from build123d import *

# Parameters (mm, degrees)
SKIZZE1_W                        = 17
SKIZZE1_H                        = 17
SKIZZE1_W_2                      = 16
SKIZZE1_H_2                      = 16
AUFSATZ_LINEAR_AUSTRAGEN1_DEPTH  = 19.7
SKIZZE10_W                       = 13.3
SKIZZE10_H                       = 20
AUFSATZ_LINEAR_AUSTRAGEN5_DEPTH  = 0.5
SKIZZE11_W                       = 5.3
SKIZZE11_H                       = 13.320508076
SCHNITT_LINEAR_AUSTRAGEN14_DEPTH = 11.433012702
AUFSATZ_LINEAR_AUSTRAGEN6_DEPTH  = 4
AUFSATZ_LINEAR_AUSTRAGEN7_DEPTH  = 4


with BuildPart() as part:
    # Skizze1 → Aufsatz-Linear austragen1 (new body)
    with BuildSketch(Plane(origin=(0, 0, 0), x_dir=(1, 0, 0), z_dir=(0, 1, 0))):
        Rectangle(SKIZZE1_W, SKIZZE1_H)
        Rectangle(SKIZZE1_W_2, SKIZZE1_H_2, mode=Mode.SUBTRACT)
    extrude(amount=AUFSATZ_LINEAR_AUSTRAGEN1_DEPTH)

    # Skizze10 → Aufsatz-Linear austragen5 (add)
    with BuildSketch(Plane(origin=(-2.530350227, 1.460898385, 0), x_dir=(0, 0, -1), z_dir=(0.866025404, -0.5, 0))):
        with Locations((-0.00194728, 31.060700455)):
            Rectangle(SKIZZE10_W, SKIZZE10_H)
    aufsatz_linear_austragen5 = extrude(amount=AUFSATZ_LINEAR_AUSTRAGEN5_DEPTH)

    # Skizze11 → Schnitt-Linear austragen14 (cut, through all)
    with BuildSketch(Plane.ZY.offset(-8)):
        with Locations((0.00194728, 26.360254038)):
            Rectangle(SKIZZE11_W, SKIZZE11_H)
    schnitt_linear_austragen14 = extrude(amount=-SCHNITT_LINEAR_AUSTRAGEN14_DEPTH, mode=Mode.SUBTRACT)

    # Skizze12 → Aufsatz-Linear austragen6 (add)
    with BuildSketch(Plane.XY.offset(6.65194728)):
        Polygon((18.433012702, 36.770508076), (8.5, 0), (8.5, 19.7), align=None)
    aufsatz_linear_austragen6 = extrude(amount=-AUFSATZ_LINEAR_AUSTRAGEN6_DEPTH)

    # Skizze13 → Aufsatz-Linear austragen7 (add)
    with BuildSketch(Plane(origin=(0, 0, -6.64805272), x_dir=(-1, 0, 0), z_dir=(0, 0, -1))):
        Polygon((-18.433012702, 36.770508076), (-8.5, 19.7), (-8.5, 0), align=None)
    aufsatz_linear_austragen7 = extrude(amount=-AUFSATZ_LINEAR_AUSTRAGEN7_DEPTH)

    # Spiegeln6: Aufsatz-Linear austragen5, Schnitt-Linear austragen14, Aufsatz-Linear austragen6, Aufsatz-Linear austragen7 across plane
    add(aufsatz_linear_austragen5.mirror(Plane(origin=(0, 0, 0), x_dir=(0, 0, 1), z_dir=(1, 0, 0))))
    add(schnitt_linear_austragen14.mirror(Plane(origin=(0, 0, 0), x_dir=(0, 0, 1), z_dir=(1, 0, 0))), mode=Mode.SUBTRACT)
    add(aufsatz_linear_austragen6.mirror(Plane(origin=(0, 0, 0), x_dir=(0, 0, 1), z_dir=(1, 0, 0))))
    add(aufsatz_linear_austragen7.mirror(Plane(origin=(0, 0, 0), x_dir=(0, 0, 1), z_dir=(1, 0, 0))))


solid = part.part
For this review, take the finished solid that the model builds, in its own axes (mm). A direction names the side the tool comes from. Give positions to 0.01 mm unless a question says otherwise; leave off trailing zeros. Order: outer loops, then holes, each group sorted by start corner. A loop starts at its lowest first (then second) coordinate and runs counter-clockwise, first axis right, second up. Notation, with made-up numbers: (54, -25.5) -> (102, -25.5) arc R19 cw to (102, -12.5) -> close; hole circle Ø1 at (-32.5, -18.5). An arc over 180 degrees is marked (long way). Write item = value, one per line.
1) We need section B-B, the plane z = -5. Give the boundary of the cut face in (x, y).
Findings:
outline = (-18.43, 36.77) -> (-8.5, 0) -> (-8, 0) -> (-8, 19.7) -> (-18, 37.02) -> close; (8, 0) -> (8.5, 0) -> (18.43, 36.77) -> (18, 37.02) -> (8, 19.7) -> close
2) Insertion check: pin 1 (6 mm diameter, centred on x = -8.5, y = 23, fed in from -Z); pin 2 (10 mm diameter, centred on y = 7, z = 5, fed in from -X); pin 3 (0.6 mm diameter, centred on x = 8.5, z = 0, fed in from +Y). Each pin has a flat end and moves straight along its axis. Give the tip position at first contact, or say it passes through.
Findings:
pin_1 = -6.65
pin_2 = -11.74
pin_3 = 19.7
3) We need section A-A, the plane z = -2. Give the boundary of the cut face in (x, y), and give its area (3 significant figures).
Findings:
outline = (-18.43, 36.77) -> (-16.27, 33.02) -> (-15.69, 33.02) -> (-18, 37.02) -> close; (-8.58, 19.7) -> (-8.5, 19.57) -> (-8.5, 0) -> (-8, 0) -> (-8, 19.7) -> close; (8, 0) -> (8.5, 0) -> (8.5, 19.57) -> (8.58, 19.7) -> (8, 19.7) -> close; (15.69, 33.02) -> (16.27, 33.02) -> (18.43, 36.77) -> (18, 37.02) -> close
area = 24.2 mm^2
4) We need section C-C, the plane x = -3.5. Give the boundary of the cut face in (y, z).
Findings:
outline = (0, -8.5) -> (19.7, -8.5) -> (19.7, -8) -> (0, -8) -> close; (0, 8) -> (19.7, 8) -> (19.7, 8.5) -> (0, 8.5) -> close
5) To check wall thickness, follow L1, parallel to Z at x = 7, y = 17; L2, parallel to Z at x = -12, y = 23.5. State the ranges of each line that lie inside material, in increasing order. Write a range as from..to.
Findings:
L1 = -8.5..-8, 8..8.5
L2 = -6.65..-2.65, 2.65..6.65
6) We need section D-D, the plane y = 27.5. Give the boundary of the cut face in (x, z).
Findings:
outline = (-15.93, -6.65) -> (-12.5, -6.65) -> (-12.5, -2.65) -> (-15.93, -2.65) -> close; (-15.93, 2.65) -> (-12.5, 2.65) -> (-12.5, 6.65) -> (-15.93, 6.65) -> close; (12.5, -6.65) -> (15.93, -6.65) -> (15.93, -2.65) -> (12.5, -2.65) -> close; (12.5, 2.65) -> (15.93, 2.65) -> (15.93, 6.65) -> (12.5, 6.65) -> close
7) For faces 5 (the face through (8.5, 10, 0)), 6 (the face through (8, 10, 0)), 7 (the face through (13.07, 28.48, 3.05)), 8 (the face through (-8.5, 10, -8)), list the 3-axis set-ups (+Z, -Z, +X, -X, +Y, -Y) from which the entire face can be reached by the end or side of a thin tool; tool diameter is ignored.
Findings:
face_5 = +X, -Y
face_6 = +Y, -Y
face_7 = +Z, -Z, +Y
face_8 = -Z, -X, +Y, -Y
8) Draft analysis for pull direction Z (two halves, no side actions). For faces 1 (the face through (-13.397, 18.128, -4.676)), 2 (the face through (-17.366, 34.922, 0.039)), 3 (the face through (0, 10, 8.5)), 4 (the face through (13, 20, 2.652)), state which applies: pulls with the +Z half, pulls with the -Z half, needs draft (parallel to the pull), parting line crosses it, or undercut.
Findings:
face_1 = needs draft
face_2 = undercut
face_3 = pulls with the +Z half
face_4 = undercut
